Input: dimensioned drawing with shaded views. Units: mm. Origin: part minimum x, y, z. A direction names the side the tool comes from. Round coordinates to 2 decimals unless told otherwise and drop trailing zeros. Loops run counter-clockwise (first coordinate to the right, second up) from the corner with the lowest first, then second, coordinate; pieces in that order, holes last. Notation, with made-up numbers: M 8.5,-35.75 L 12.5,-35.75 A13 ccw 12.5,-23.75 Z; hole C 0.25,57 d2. An arc over 180 degrees is marked long. One line per item, written item: value.
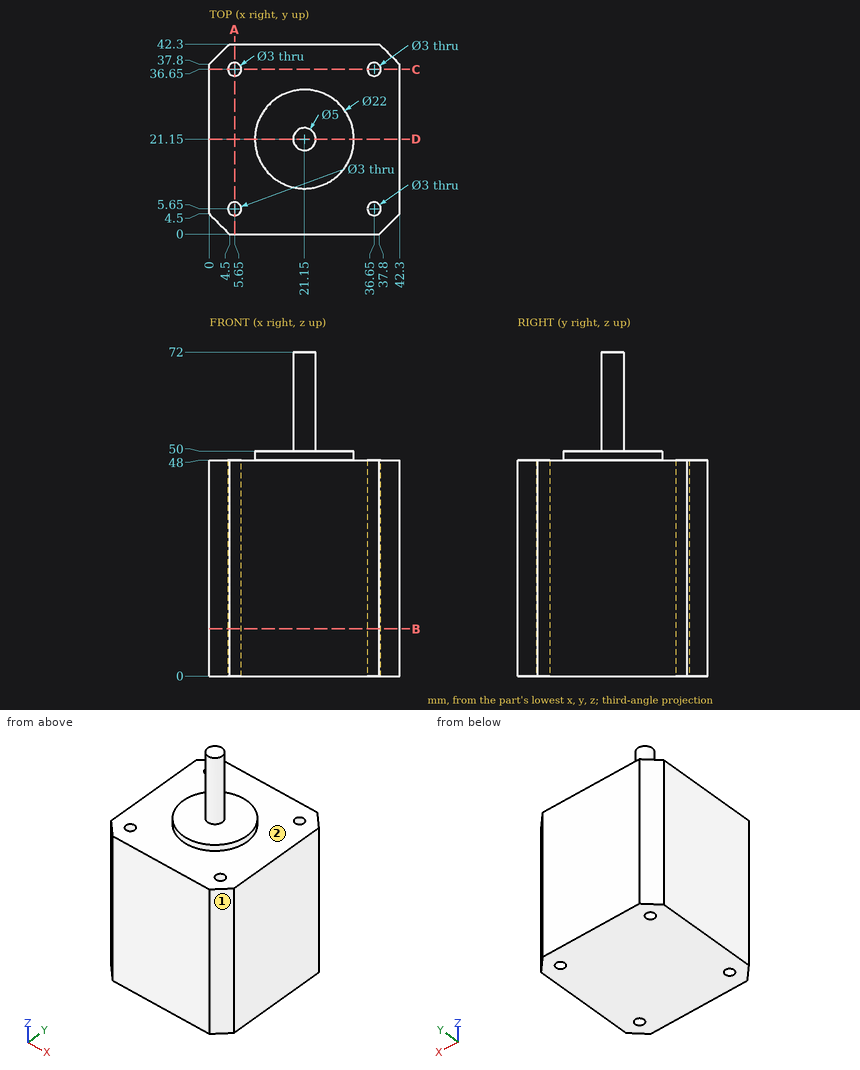
1. Section query B-B (z = 10.5). Return the cut outline in (x, y).
Report:
outline: M 0,4.5 L 4.5,0 L 37.8,0 L 42.3,4.5 L 42.3,37.8 L 37.8,42.3 L 4.5,42.3 L 0,37.8 Z; hole C 5.65,5.65 d3; hole C 5.65,36.65 d3; hole C 36.65,5.65 d3; hole C 36.65,36.65 d3
2. Pin query (flat end, axial travel): pin 1 (4 mm diameter, centred on x = 24, y = 9, fed in from +Z); pin 2 (1 mm diameter, centred on y = 22, z = 64.5, fed in from -X). Return the tip coordinate at first contact, or that it passes through.
Report:
pin 1: stops at z = 50
pin 2: stops at x = 18.67
3. Section query D-D (y = 21.15). Return the cut outline in (x, z), and give its area (3 significant figures).
Report:
outline: M 0,0 L 42.3,0 L 42.3,48 L 32.15,48 L 32.15,50 L 23.65,50 L 23.65,72 L 18.65,72 L 18.65,50 L 10.15,50 L 10.15,48 L 0,48 Z
area: 2,180 mm2
4. Ray query, line 1 (X direction, y = 36.5, z = 42); line 2 (Y direction, x = 5.65, z = 15.5); line 3 (Y direction, x = 5, z = 18). Return the intervals inside material, ascending. Write a range as [from, to].
Report:
line 1: x = [0, 4.16], [7.14, 35.16], [38.14, 42.3]
line 2: y = [0, 4.15], [7.15, 35.15], [38.15, 42.3]
line 3: y = [0, 4.3], [7, 35.3], [38, 42.3]
5. Reachability of the marked faces 1 and 2 from +Z, -Z, +X, -X, +Y, -Y: full face, straight path, thin tool, end or side. Return the list, or none.
Report:
face 1: +Z, -Z, +X, -Y
face 2: +Z
6. Section query A-A (x = 5.65). Return the cut outline in (y, z), and give its area (3 significant figures).
Report:
outline: M 0,0 L 4.15,0 L 4.15,48 L 0,48 Z; M 7.15,0 L 35.15,0 L 35.15,48 L 7.15,48 Z; M 38.15,0 L 42.3,0 L 42.3,48 L 38.15,48 Z
area: 1,740 mm2
